Input: part model. Units: mm. Frame: model coordinates. Face numbers are marked on the shaded views. A direction names the side the tool comes from. Give positions to 0.01 mm unless a question says otherwise; leave off trailing zeros. Loops run counter-clockwise (first coordinate to the right, second up) from the corner with the lowest first, then second, coordinate; pieces in that order, holes last. Notation, with made-up numbers: (49, 57) - (60, 57) arc R25 cw to (60, 89) - close; hole circle Ø6 at (61, 25). An arc over 180 degrees is marked (long way). Answer as a JSON object with one key per item and string values. Group by question number.
(1) Section query D-D (y = 5). Return loops of the section in (x, z), plus the area to 3 significant figures.
(2) Material intervals for L1, parallel to Y at x = 20.5, z = 26.25; L2, parallel to X at y = 59, z = 22; L3, parallel to X at y = 50, z = 11, sorted ascending.
(3) Mould query, pull axis X, two halves, no side actions, for the marked faces 6, 7, 8 and 9. Classes: +X half, -X half, draft (parallel to the pull), parting line (faces both ways), or undercut.
(4) Access query for the marked faces 1, 2, 3, 4 and 5. Directions: +Z, -Z, +X, -X, +Y, -Y. A direction counts if a zero-diameter tool reaches every point of the face in a straight line with its end or side. Return the directions, or none.
(5) Section query C-C (x = 20.5). Return loops of the section in (y, z).
(6) Section query A-A (z = 9.5). Return loops of the section in (x, y).
(7) Pin query (flat end, axial travel): P1, Ø2, axis at y = 16, z = 6.5, coming from the -X side; P2, Ø3, axis at x = 1.5, z = 13.5, coming from the -Y side; P3, Ø1, axis at x = 26.5, z = 21.5, coming from the +Y side; P4, Ø8, axis at y = 12.5, z = 0.5, coming from the -X side. Return the tip coordinate at first contact, or that it passes through.
(8) Section query B-B (y = 26). Return loops of the section in (x, z).
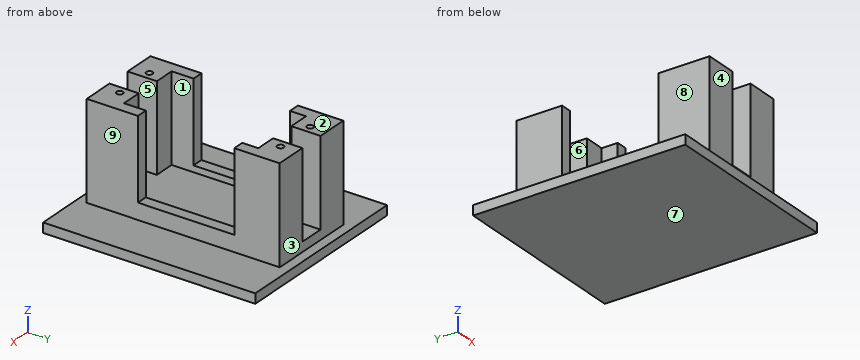
```python
from build123d import *

# Parameters (mm, degrees)
SKETCH_W        = 28
SKETCH_H        = 60
PAD_DEPTH       = 30
SKETCH001_W     = 21
SKETCH001_H     = 41.8
POCKET_DEPTH    = 27
SKETCH002_W     = 3.5
SKETCH002_H     = 30
POCKET001_DEPTH = 25
SKETCH003_W     = 3.5
SKETCH003_H     = 30
POCKET002_DEPTH = 25
SKETCH006_W     = 8
SKETCH006_H     = 7
POCKET005_DEPTH = 60.001
SKETCH007_R     = 1
POCKET006_DEPTH = 7
SKETCH008_R     = 1
POCKET007_DEPTH = 7
SKETCH009_W     = 8
SKETCH009_H     = 20
POCKET008_DEPTH = 60.001
SKETCH010_W     = 58
SKETCH010_H     = 60
PAD001_DEPTH    = 3
SKETCH011_W     = 58
SKETCH011_H     = 3
PAD002_DEPTH    = 3
SKETCH012_W     = 58
SKETCH012_H     = 3
PAD003_DEPTH    = 3


with BuildPart() as part:
    # Sketch → Pad (new body)
    with BuildSketch(Plane.XY):
        with Locations((14, 30)):
            Rectangle(SKETCH_W, SKETCH_H)
    extrude(amount=PAD_DEPTH)

    # Sketch001 (on Face6 of Pad) → Pocket (cut)
    with BuildSketch(Plane.XY.offset(30)):
        with Locations((14, 30)):
            Rectangle(SKETCH001_W, SKETCH001_H)
    extrude(amount=-POCKET_DEPTH, mode=Mode.SUBTRACT)

    # Sketch002 (on Face5 of Pocket) → Pocket001 (cut)
    with BuildSketch(Plane.XY.offset(30)):
        with Locations((1.75, 30.9)):
            Rectangle(SKETCH002_W, SKETCH002_H)
    extrude(amount=-POCKET001_DEPTH, mode=Mode.SUBTRACT)

    # Sketch003 (on Face5 of Pocket) → Pocket002 (cut)
    with BuildSketch(Plane.XY.offset(30)):
        with Locations((26.25, 30.9)):
            Rectangle(SKETCH003_W, SKETCH003_H)
    extrude(amount=-POCKET002_DEPTH, mode=Mode.SUBTRACT)

    # Sketch006 → Pocket005 (cut, through all)
    with BuildSketch(Plane(origin=(0, 60, 0), x_dir=(-1, 0, 0), z_dir=(0, 1, 0))):
        with Locations((-14, 6.5)):
            Rectangle(SKETCH006_W, SKETCH006_H)
    extrude(amount=-POCKET005_DEPTH, mode=Mode.SUBTRACT)

    # Sketch007 (on Face4 of Pocket005) → Pocket006 (cut)
    with BuildSketch(Plane.XY.offset(30)):
        with Locations((7.5, 5)):
            Circle(SKETCH007_R)
        with Locations((20.5, 5)):
            Circle(SKETCH007_R)
    extrude(amount=-POCKET006_DEPTH, mode=Mode.SUBTRACT)

    # Sketch008 (on Face13 of Pocket005) → Pocket007 (cut)
    with BuildSketch(Plane.XY.offset(30)):
        with Locations((7.5, 55)):
            Circle(SKETCH008_R)
        with Locations((20.5, 55)):
            Circle(SKETCH008_R)
    extrude(amount=-POCKET007_DEPTH, mode=Mode.SUBTRACT)

    # Sketch009 (on Face1 of Pocket007) → Pocket008 (cut, through all)
    with BuildSketch(Plane.XZ):
        with Locations((14, 20)):
            Rectangle(SKETCH009_W, SKETCH009_H)
    extrude(amount=-POCKET008_DEPTH, mode=Mode.SUBTRACT)

    # Sketch010 (on Face2 of Pocket008) → Pad001 (join)
    with BuildSketch(Plane(origin=(0, 0, 0), x_dir=(1, 0, 0), z_dir=(0, 0, -1))):
        with Locations((14, -30)):
            Rectangle(SKETCH010_W, SKETCH010_H)
    extrude(amount=PAD001_DEPTH)

    # Sketch011 (on Face1 of Pad001) → Pad002 (join)
    with BuildSketch(Plane.XZ):
        with Locations((14, -1.5)):
            Rectangle(SKETCH011_W, SKETCH011_H)
    extrude(amount=PAD002_DEPTH)

    # Sketch012 (on Face8 of Pad001) → Pad003 (join)
    with BuildSketch(Plane(origin=(0, 60, 0), x_dir=(-1, 0, 0), z_dir=(0, 1, 0))):
        with Locations((-14, -1.5)):
            Rectangle(SKETCH012_W, SKETCH012_H)
    extrude(amount=PAD003_DEPTH)


solid = part.part
```
Recorded:
{
 "1": {"outline": "(-15, -3) - (43, -3) - (43, 0) - (28, 0) - (28, 30) - (21.5, 30) - (21.5, 23) - (19.5, 23) - (19.5, 30) - (18, 30) - (18, 3) - (10, 3) - (10, 30) - (8.5, 30) - (8.5, 23) - (6.5, 23) - (6.5, 30) - (0, 30) - (0, 0) - (-15, 0) - close", "area": "770 mm^2"},
 "2": {"L1": "y = 0 to 4, 6 to 9.1, 50.9 to 54, 56 to 60", "L2": "x = 0 to 10, 18 to 28", "L3": "x = 0 to 3.5, 24.5 to 28"},
 "3": {"face 6": "undercut", "face 7": "draft", "face 8": "-X half", "face 9": "+X half"},
 "4": {"face 1": "+Z", "face 2": "+Z, +X, -X, +Y, -Y", "face 3": "+Z, +X, -X, +Y", "face 4": "+Z, +X, -X, -Y", "face 5": "+Z, +Y, -Y"},
 "5": {"outline": "(-3, -3) - (63, -3) - (63, 0) - (60, 0) - (60, 30) - (56, 30) - (56, 23) - (54, 23) - (54, 30) - (50.9, 30) - (50.9, 3) - (9.1, 3) - (9.1, 30) - (6, 30) - (6, 23) - (4, 23) - (4, 30) - (0, 30) - (0, 0) - (-3, 0) - close"},
 "6": {"outline": "(0, 0) - (10, 0) - (10, 9.1) - (3.5, 9.1) - (3.5, 15.9) - (0, 15.9) - close; (0, 45.9) - (3.5, 45.9) - (3.5, 50.9) - (10, 50.9) - (10, 60) - (0, 60) - close; (18, 0) - (28, 0) - (28, 15.9) - (24.5, 15.9) - (24.5, 9.1) - (18, 9.1) - close; (18, 50.9) - (24.5, 50.9) - (24.5, 45.9) - (28, 45.9) - (28, 60) - (18, 60) - close"},
 "7": {"P1": "stops at x = 0", "P2": "stops at y = 0", "P3": "stops at y = 60", "P4": "stops at x = -15"},
 "8": {"outline": "(-15, -3) - (43, -3) - (43, 0) - (28, 0) - (28, 5) - (24.5, 5) - (24.5, 3) - (3.5, 3) - (3.5, 5) - (0, 5) - (0, 0) - (-15, 0) - close"}
}
